```python
from build123d import *

# Parameters (mm, degrees)
SKETCH_1_W          = 36
SKETCH_1_H          = 30
EXTRUDE_1_DEPTH     = 12
SKETCH_2_R          = 2.5
CUT_EXTRUDE_2_DEPTH = 12
SKETCH_3_R          = 2.5
CUT_EXTRUDE_3_DEPTH = 12


with BuildPart() as part:
    # 草图1 → 凸台-拉伸1 (new body)
    with BuildSketch(Plane.XY):
        Rectangle(SKETCH_1_W, SKETCH_1_H)
    extrude(amount=EXTRUDE_1_DEPTH)

    # 草图2 → 切除-拉伸2 (cut)
    with BuildSketch(Plane.XY.offset(12)):
        with Locations((-12, 5)):
            Circle(SKETCH_2_R)
        with Locations((12, 5)):
            Circle(SKETCH_2_R)
        with Locations((12, -10)):
            Circle(SKETCH_2_R)
        with Locations((-12, -10)):
            Circle(SKETCH_2_R)
    extrude(amount=-CUT_EXTRUDE_2_DEPTH, mode=Mode.SUBTRACT)

    # 草图3 → 切除-拉伸3 (cut)
    with BuildSketch(Plane.XY.offset(12)):
        with Locations((0, 10)):
            Circle(SKETCH_3_R)
    extrude(amount=-CUT_EXTRUDE_3_DEPTH, mode=Mode.SUBTRACT)


solid = part.part
```
The model under review builds one solid part; all positions refer to its coordinate system, in mm. Give positions to 0.01 mm unless a question says otherwise; leave off trailing zeros. Write each loop counter-clockwise with the first axis right and the second up, starting at its lowest first coordinate (ties: lowest second). Pieces come first, ordered by that corner, then holes. Notation, with made-up numbers: M 87.25,-28.5 L 105.25,-28.5 A37 cw 105.25,10.5 Z; hole C 0,11.25 d8. An arc over 180 degrees is marked long. Write each question's results on one line, items separated by ' | '. Start each with the question number.
1. We need section C-C (z = 8.75). Write out the cut boundary in (x, y), and give its area (3 significant figures).
2. We need section D-D (x = -1.5). Write out the cut boundary in (y, z), and give its area (3 significant figures).
3. For probe 1 along Y at (x, z) = (-12, 2.5); probe 2 along X at (y, z) = (-11.5, 7.5); probe 3 along Y at (x, z) = (-13.5, 10.5), list the stretches that pass through material, from the lowest coordinate up. Write a range as [from, to].
4. We need section B-B (y = 5). Write out the cut boundary in (x, z), and give its area (3 significant figures).
5. We need section A-A (x = -12). Write out the cut boundary in (y, z).
6. Mouldability with a two-part tool opening along X and no side actions: class faces 1 (the cylindrical face through (-0.54, 7.56, 6.08)), 2 (the flat face through (0, 0, 0)), 3 (the flat face through (18, 0, 6)) as released by +X, released by -X, zero draft, split by the parting line, or undercut.
Results found:
1) outline: M -18,-15 L 18,-15 L 18,15 L -18,15 Z; hole C -12,-10 d5; hole C -12,5 d5; hole C 0,10 d5; hole C 12,-10 d5; hole C 12,5 d5 | area: 982 mm^2
2) outline: M -15,0 L 8,0 L 8,12 L -15,12 Z; M 12,0 L 15,0 L 15,12 L 12,12 Z | area: 312 mm^2
3) probe 1: y = [-15, -12.5], [-7.5, 2.5], [7.5, 15] | probe 2: x = [-18, -14], [-10, 10], [14, 18] | probe 3: y = [-15, -12], [-8, 3], [7, 15]
4) outline: M -18,0 L -14.5,0 L -14.5,12 L -18,12 Z; M -9.5,0 L 9.5,0 L 9.5,12 L -9.5,12 Z; M 14.5,0 L 18,0 L 18,12 L 14.5,12 Z | area: 312 mm^2
5) outline: M -15,0 L -12.5,0 L -12.5,12 L -15,12 Z; M -7.5,0 L 2.5,0 L 2.5,12 L -7.5,12 Z; M 7.5,0 L 15,0 L 15,12 L 7.5,12 Z
6) face 1: undercut | face 2: zero draft | face 3: released by +X
